Check sheet for the modelled part. Datum: model origin and axes. Units: mm. Coordinates: 2 decimals unless noted, no trailing zeros. Loops run counter-clockwise (first coordinate to the right, second up) from the corner with the lowest first, then second, coordinate; pieces in that order, holes last. Notation, with made-up numbers: (86, 57.25) -> (94, 57.25) arc R12 cw to (94, 80.25) -> close; hole circle Ø5 at (39, 73.25). An arc over 180 degrees is marked (long way). Use one line per item in the form item = value.
from build123d import *

# Parameters (mm, degrees)
SKETCH1_W           = 110
SKETCH1_H           = 60
BOSS_EXTRUDE1_DEPTH = 3.175
SKETCH2_R           = 3.25
CUT_EXTRUDE1_DEPTH  = 4.175
FILLET1_R           = 10


with BuildPart() as part:
    # Sketch1 → Boss-Extrude1 (new body)
    with BuildSketch(Plane.XY):
        Rectangle(SKETCH1_W, SKETCH1_H)
    extrude(amount=BOSS_EXTRUDE1_DEPTH)

    # Sketch2 → Cut-Extrude1 (cut, through all)
    with BuildSketch(Plane.XY.offset(3.175)):
        with Locations((-40, 20)):
            Circle(SKETCH2_R)
        with Locations((40, 20)):
            Circle(SKETCH2_R)
        with Locations((-20, 20)):
            Circle(SKETCH2_R)
        with Locations((0, 20)):
            Circle(SKETCH2_R)
        with Locations((20, 20)):
            Circle(SKETCH2_R)
        with Locations((44.66, -15)):
            Circle(SKETCH2_R)
        with Locations((5, -20)):
            Circle(SKETCH2_R)
        with Locations((0, -10)):
            Circle(SKETCH2_R)
        with Locations((-5, -20)):
            Circle(SKETCH2_R)
        with Locations((-10, -10)):
            Circle(SKETCH2_R)
        with Locations((-15, -20)):
            Circle(SKETCH2_R)
        with Locations((10, -10)):
            Circle(SKETCH2_R)
        with Locations((-20, -10)):
            Circle(SKETCH2_R)
        with Locations((-44.66, -15)):
            Circle(SKETCH2_R)
        with Locations((20, -10)):
            Circle(SKETCH2_R)
        with Locations((15, -20)):
            Circle(SKETCH2_R)
        with Locations((-25, -20)):
            Circle(SKETCH2_R)
        with Locations((25, -20)):
            Circle(SKETCH2_R)
    extrude(amount=-CUT_EXTRUDE1_DEPTH, mode=Mode.SUBTRACT)

    # Fillet1
    fillet1_edges = [part.edges().sort_by_distance(p)[0] for p in [
        (55, -30, 1.5875),
        (-55, -30, 1.5875),
        (-55, 30, 1.5875),
        (55, 30, 1.5875),
    ]]
    fillet(fillet1_edges, radius=FILLET1_R)


solid = part.part
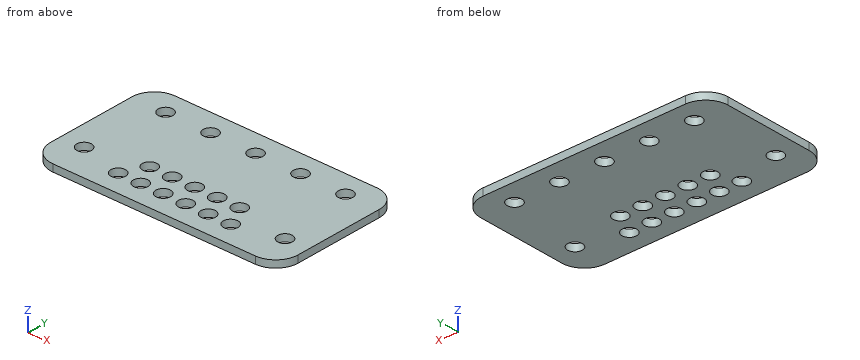
(1) Section check C-C, the plane z = 2.4. Give the number of separate pieces and of enclosed holes in the cut face, plus the area to 3 significant figures.
Established:
separate_pieces = 1
enclosed_holes = 18
area = 5,920 mm²
(2) Go/stop test with flat-tipped pins: P1, Ø7.5, axis at x = 40, y = 20, coming from the -Z side; P2, Ø5, axis at x = -10, y = -10, coming from the +Z side. Record where each tip stops, or that it passes through.
Established:
P1 = 0
P2 = through
(3) Scan lines: line 1 along Y through (x, z) = (-10, 1.3); line 2 along Y through (x, z) = (15, 1.1); line 3 along Y through (x, z) = (-8, 2.3). Record each from-to range of solid material in increasing order.
Established:
line_1 = -30 to -13.25, -6.75 to 30
line_2 = -30 to -23.25, -16.75 to 30
line_3 = -30 to -21.25, -18.75 to -12.56, -7.44 to 30
(4) Section check D-D, the plane x = 5. Record the boundary of the cut face in (y, z) (3 decimals).
Established:
outline = (-30, 0) -> (-23.25, 0) -> (-23.25, 3.175) -> (-30, 3.175) -> close; (-16.75, 0) -> (30, 0) -> (30, 3.175) -> (-16.75, 3.175) -> close
(5) Section check A-A, the plane y = -15. Record the boundary of the cut face in (x, z) (3 decimals).
Established:
outline = (-55, 0) -> (-47.91, 0) -> (-47.91, 3.175) -> (-55, 3.175) -> close; (-41.41, 0) -> (41.41, 0) -> (41.41, 3.175) -> (-41.41, 3.175) -> close; (47.91, 0) -> (55, 0) -> (55, 3.175) -> (47.91, 3.175) -> close
(6) Section check B-B, the plane x = -20. Record the boundary of the cut face in (y, z) (3 decimals).
Established:
outline = (-30, 0) -> (-13.25, 0) -> (-13.25, 3.175) -> (-30, 3.175) -> close; (-6.75, 0) -> (16.75, 0) -> (16.75, 3.175) -> (-6.75, 3.175) -> close; (23.25, 0) -> (30, 0) -> (30, 3.175) -> (23.25, 3.175) -> close
